Here's how the part is built. I have some questions about the finished solid (model axes, mm). Coordinates: 2 decimals unless noted, no trailing zeros. Write each loop counter-clockwise with the first axis right and the second up, starting at its lowest first coordinate (ties: lowest second). Pieces come first, ordered by that corner, then holes. Notation, with made-up numbers: (70, 24) - (108, 24) arc R34 cw to (108, 55) - close; hole circle Ø4 at (-8.75, 1). An arc over 180 degrees is marked (long way). Answer in a Markdown table with one row per item. Add a question column.
Item 1: Imagine slicing it at C-C (x = 256). Please give me the cut outline in (y, z), plus the area to 3 significant figures.
Item 2: Imagine slicing it at A-A (y = 0.6). State how many separate pieces and enclosed holes the cut face has, plus the area to 3 significant figures.
Item 3: Imagine slicing it at B-B (z = -20.5). Please give me the cut outline in (x, y), plus the area to 3 significant figures.
Item 4: If I drill on probe 1 along X at (y, z) = (0.6, 0); probe 2 along Z at (x, y) = (187.96, 0.65); probe 3 along Z at (x, y) = (238.76, 0.4), over which ranges is the centre line in solid material (lowest first)? Write a range as from..to.
Item 5: I'm going to push a flat-ended pin straight in: pin 1 (1.3 mm diameter, centred on x = -36.195, z = 0, fed in from +Y). Where does the tip first touch, or does it pass through?
from build123d import *

# Parameters (mm, degrees)
SKETCH1_R           = 1.0922
SKETCH1_R_2         = 2.1
BOSS_EXTRUDE1_DEPTH = 1.5875


with BuildPart() as part:
    # Sketch1 → Boss-Extrude1 (new body)
    with BuildSketch(Plane(origin=(0, 0, 0), x_dir=(1, 0, 0), z_dir=(0, 1, 0))):
        with BuildLine():
            Line((0, 39.37), (238.76, 39.37))
            ThreePointArc((238.76, 39.37), (278.13, 0), (238.76, -39.37))
            Line((238.76, -39.37), (0, -39.37))
            ThreePointArc((0, -39.37), (-39.37, 0), (0, 39.37))
        make_face()
        with Locations((50.8, 36.195)):
            Circle(SKETCH1_R, mode=Mode.SUBTRACT)
        with Locations((187.96, 36.195)):
            Circle(SKETCH1_R, mode=Mode.SUBTRACT)
        with Locations((50.8, -36.195)):
            Circle(SKETCH1_R, mode=Mode.SUBTRACT)
        with Locations((187.96, -36.195)):
            Circle(SKETCH1_R, mode=Mode.SUBTRACT)
        with Locations((-36.195, 0)):
            Circle(SKETCH1_R, mode=Mode.SUBTRACT)
        with Locations((276.5425, 0)):
            Circle(SKETCH1_R, mode=Mode.SUBTRACT)
        with Locations((238.76, 0)):
            Circle(SKETCH1_R_2, mode=Mode.SUBTRACT)
        with Locations((0, -6.35)):
            Circle(SKETCH1_R_2, mode=Mode.SUBTRACT)
        with Locations((0, 6.35)):
            Circle(SKETCH1_R_2, mode=Mode.SUBTRACT)
    extrude(amount=BOSS_EXTRUDE1_DEPTH)


solid = part.part
Here are the results:
| question | item | result |
|---|---|---|
| 1 | outline | (0, -35.39) - (1.59, -35.39) - (1.59, 35.39) - (0, 35.39) - close |
| 1 | area | 112 mm2 |
| 2 | separate pieces | 1 |
| 2 | enclosed holes | 9 |
| 2 | area | 23,600 mm2 |
| 3 | outline | (-33.61, 0) - (272.37, 0) - (272.37, 1.59) - (-33.61, 1.59) - close |
| 3 | area | 486 mm2 |
| 4 | probe 1 | x = -39.37..-37.29, -35.1..236.66, 240.86..275.45, 277.63..278.13 |
| 4 | probe 2 | z = -39.37..-37.29, -35.1..35.1, 37.29..39.37 |
| 4 | probe 3 | z = -39.37..-2.1, 2.1..39.37 |
| 5 | pin 1 | passes through |
